Could you check a few things on this model? Use its own coordinates, in mm. A direction names the side the tool comes from. Coordinates: 2 decimals unless noted, no trailing zeros. Write each loop counter-clockwise with the first axis right and the second up, starting at its lowest first coordinate (ties: lowest second). Pieces come first, ordered by that corner, then holes. Notation, with made-up numbers: M 16,-36 L 75,-36 A27 ccw 75,-2 Z; hole C -11,-33.75 d11. An arc over 180 degrees is marked long. Answer as CSV lines item,"result". Start each with the question number.
Item 1: If I drill on line 1 along Y through (x, z) = (-2, 0.2); line 2 along X through (y, z) = (-6.5, 1.15); line 3 along X through (y, z) = (-9.75, 0.25), over which ranges is the centre line in solid material (lowest first)? Write a range as [from, to].
Item 2: Suppose I cut it at B-B, the plane z = 1.3. Write out the boundary of the cut face in (x, y).
Item 3: I'm going to push a flat-ended pin straight in: P1, Ø1, axis at x = 21, z = 2, coming from the -Y side. Where does the tip first touch, or does it pass through?
Item 4: Suppose I cut it at A-A, the plane y = -10.5. Write out the boundary of the cut face in (x, z).
Item 5: We'd pull the mould along X, two halves only. Please class faces 3 (the flat face through (0, 0, 3)), 4 (the flat face through (0, -6.25, 2)): +X half, -X half, draft (parallel to the pull), parting line (faces both ways), or undercut.
Item 6: Suppose I cut it at D-D, the plane x = 14. Write out the boundary of the cut face in (y, z).
Item 7: Suppose I cut it at C-C, the plane x = 7.5. Write out the boundary of the cut face in (y, z), and give its area (3 significant figures).
Item 8: On a 3-axis mill with a long thin cutter (end or side, diameter ignored), from which of +Z, -Z, +X, -X, +Y, -Y can I reach the whole of each face in a straight line? I mean faces 1 (the flat face through (0, 6.25, 2)), 2 (the flat face through (0, 0, 0)). Say none if no direction works.
```python
from build123d import *

# Parameters (mm, degrees)
ESQUISSE1_W             = 60
ESQUISSE1_H             = 25
BOSS_EXTRU_2_DEPTH      = 3
ENL_V_MAT_EXTRU_1_DEPTH = 10


with BuildPart() as part:
    # Esquisse1 → Boss.-Extru.2 (new body)
    with BuildSketch(Plane.XY):
        Rectangle(ESQUISSE1_W, ESQUISSE1_H)
    extrude(amount=BOSS_EXTRU_2_DEPTH)

    # Esquisse2 → Enlèv. mat.-Extru.1 (cut)
    with BuildSketch(Plane.XY.offset(3)):
        with BuildLine():
            Line((-6.674682453, 6.25), (0, 6.25))
            Line((0, 6.25), (6.674682453, 6.25))
            ThreePointArc((6.674682453, 6.25), (11.249999964, 10.825317527), (17.499999917, 12.5))
            Line((17.499999917, 12.5), (-17.500000011, 12.5))
            ThreePointArc((-17.500000011, 12.5), (-11.250000005, 10.82531755), (-6.674682453, 6.25))
        make_face()
        with BuildLine():
            ThreePointArc((-30, 3e-08), (-26.338834758, 8.838834771), (-17.500000011, 12.5))
            Line((-17.500000011, 12.5), (-30, 12.5))
            Line((-30, 12.5), (-30, 3e-08))
        make_face()
        with BuildLine():
            Line((-30, -12.5), (-17.50000003, -12.5))
            ThreePointArc((-17.50000003, -12.5), (-26.338834786, -8.838834744), (-30, 3e-08))
            Line((-30, 3e-08), (-30, -12.5))
        make_face()
        with BuildLine():
            Line((6.674682453, -6.25), (0, -6.25))
            Line((0, -6.25), (-6.674682453, -6.25))
            ThreePointArc((-6.674682453, -6.25), (-11.250000013, -10.825317555), (-17.50000003, -12.5))
            Line((-17.50000003, -12.5), (17.500000079, -12.5))
            ThreePointArc((17.500000079, -12.5), (11.250000034, -10.825317567), (6.674682453, -6.25))
        make_face()
        with BuildLine():
            ThreePointArc((30, -1.2e-08), (26.338834789, -8.838834741), (17.500000079, -12.5))
            Line((17.500000079, -12.5), (30, -12.5))
            Line((30, -12.5), (30, -1.2e-08))
        make_face()
        with BuildLine():
            Line((30, 12.5), (17.499999917, 12.5))
            ThreePointArc((17.499999917, 12.5), (26.33883474, 8.83883479), (30, -1.2e-08))
            Line((30, -1.2e-08), (30, 12.5))
        make_face()
    extrude(amount=-ENL_V_MAT_EXTRU_1_DEPTH, mode=Mode.SUBTRACT)


solid = part.part
```
Ans:
1,line 1,"y = [-6.25, 6.25]"
1,line 2,"x = [-28.18, -6.82], [6.82, 28.18]"
1,line 3,"x = [-25.32, -9.68], [9.68, 25.32]"
2,outline,"M -6.67,-6.25 L 6.67,-6.25 A12.5 ccw long 6.67,6.25 L -6.67,6.25 A12.5 ccw long Z"
3,P1,"stops at y = -12.13"
4,outline,"M -24.28,0 L -10.72,0 L -10.72,3 L -24.28,3 Z; M 10.72,0 L 24.28,0 L 24.28,3 L 10.72,3 Z"
5,face 3,"draft"
5,face 4,"undercut"
6,outline,"M -12,0 L 12,0 L 12,3 L -12,3 Z"
7,outline,"M -7.5,0 L 7.5,0 L 7.5,3 L -7.5,3 Z"
7,area,"45.0 mm^2"
8,face 1,"+Z, -Z, +Y"
8,face 2,"-Z, +X, -X, +Y, -Y"
